Check sheet for the modelled part. Datum: model origin and axes. Units: mm. A direction names the side the tool comes from. Coordinates: 2 decimals unless noted, no trailing zeros. Write each loop counter-clockwise with the first axis right and the second up, starting at its lowest first coordinate (ties: lowest second). Pieces come first, ordered by that corner, then holes. Notation, with made-up numbers: (81.25, 45) -> (138.25, 45) arc R13 cw to (138.25, 62) -> close; hole circle Ø7 at (-18, 47). An arc over 180 degrees is marked (long way). Put each result on its own line as item: value.
```python
from build123d import *

# Parameters (mm, degrees)
BOSS_EXTRUDE1_DEPTH = 6
SKETCH2_W           = 6
SKETCH2_H           = 25.4
SKETCH2_W_2         = 31.8008
SKETCH2_H_2         = 3.048
BOSS_EXTRUDE4_DEPTH = 6
FILLET1_R           = 3.175
KERF_DEPTH          = 6


with BuildPart() as part:
    # Sketch1 → Boss-Extrude1 (new body)
    with BuildSketch(Plane(origin=(0, 0, 0), x_dir=(1, 0, 0), z_dir=(0, 1, 0))):
        Polygon((-3.175, 76.2), (-3.175, -76.2), (57.15, -76.2), (0, 76.2), align=None)
    extrude(amount=BOSS_EXTRUDE1_DEPTH)

    # Sketch2 → Boss-Extrude4 (add)
    with BuildSketch(Plane(origin=(0, 0, 0), x_dir=(1, 0, 0), z_dir=(0, 1, 0))):
        with Locations((-6.175, 0)):
            Rectangle(SKETCH2_W, SKETCH2_H)
        with Locations((-6.175, 38.1)):
            Rectangle(SKETCH2_W, SKETCH2_H)
        with Locations((-6.175, -38.1)):
            Rectangle(SKETCH2_W, SKETCH2_H)
        with Locations((25.4, -77.724)):
            Rectangle(SKETCH2_W_2, SKETCH2_H_2)
    extrude(amount=BOSS_EXTRUDE4_DEPTH)

    # Fillet1
    fillet1_edges = [part.edges().sort_by_distance(p)[0] for p in [
        (0, 3, -76.2),
        (57.15, 3, 76.2),
    ]]
    fillet(fillet1_edges, radius=FILLET1_R)

    # Sketch3 → KERF (add)
    with BuildSketch(Plane(origin=(0, 6, 0), x_dir=(1, 0, 0), z_dir=(0, 1, 0))):
        with BuildLine():
            Line((41.402, -76.3016), (52.568473514, -76.3016))
            ThreePointArc((52.568473514, -76.3016), (55.261594992, -74.891334445), (55.636449697, -71.874508931))
            Line((55.636449697, -71.874508931), (0.867699697, 74.175491069))
            ThreePointArc((0.867699697, 74.175491069), (-0.333942041, 75.718121478), (-2.200276486, 76.3016))
            Line((-2.200276486, 76.3016), (-3.2766, 76.3016))
            Line((-3.2766, 76.3016), (-3.2766, 50.9016))
            Line((-3.2766, 50.9016), (-9.2766, 50.9016))
            Line((-9.2766, 50.9016), (-9.2766, 25.2984))
            Line((-9.2766, 25.2984), (-3.2766, 25.2984))
            Line((-3.2766, 25.2984), (-3.2766, 12.8016))
            Line((-3.2766, 12.8016), (-9.2766, 12.8016))
            Line((-9.2766, 12.8016), (-9.2766, -12.8016))
            Line((-9.2766, -12.8016), (-3.2766, -12.8016))
            Line((-3.2766, -12.8016), (-3.2766, -25.2984))
            Line((-3.2766, -25.2984), (-9.2766, -25.2984))
            Line((-9.2766, -25.2984), (-9.2766, -50.9016))
            Line((-9.2766, -50.9016), (-3.2766, -50.9016))
            Line((-3.2766, -50.9016), (-3.2766, -76.3016))
            Line((-3.2766, -76.3016), (9.398, -76.3016))
            Line((9.398, -76.3016), (9.398, -79.3496))
            Line((9.398, -79.3496), (41.402, -79.3496))
            Line((41.402, -79.3496), (41.402, -76.3016))
        make_face()
    extrude(amount=-KERF_DEPTH)


solid = part.part
```
Q1. Tool access check on faces 4 (the flat face through (9.398, 3, 78)), 5 (the cylindrical face through (-0.31, 3.04, -75.7)), 6 (the flat face through (-6, 3, 12.802)), 7 (the flat face through (41.402, 3, 78)). Record the directions out of +Z, -Z, +X, -X, +Y, -Y that give a thin tool (end or side, any length) a straight path to the whole face; none if there is none.
Recorded:
face 4: +Z, -X, +Y, -Y
face 5: -Z, +X, +Y, -Y
face 6: -X, +Y, -Y
face 7: +Z, +X, +Y, -Y
Q2. Mould release check, pull along Z, two halves, no side actions. Record for faces 1 (the flat face through (-3.277, 3, -64)), 2 (the flat face through (47, 3, 76.302)), 3 (the flat face through (-3.277, 3, -19)): released by +Z, released by -Z, zero draft, split by the parting line, or undercut.
Recorded:
face 1: zero draft
face 2: released by +Z
face 3: undercut
Q3. Cross-section at A-A (y = 2.1). Record the cut outline in (x, z) (1 decimal).
Recorded:
outline: (-9.3, -50.9) -> (-3.3, -50.9) -> (-3.3, -76.3) -> (-2.2, -76.3) arc R3.3 ccw to (0.9, -74.2) -> (55.6, 71.9) arc R3.3 ccw to (52.6, 76.3) -> (41.4, 76.3) -> (41.4, 79.3) -> (9.4, 79.3) -> (9.4, 76.3) -> (-3.3, 76.3) -> (-3.3, 50.9) -> (-9.3, 50.9) -> (-9.3, 25.3) -> (-3.3, 25.3) -> (-3.3, 12.8) -> (-9.3, 12.8) -> (-9.3, -12.8) -> (-3.3, -12.8) -> (-3.3, -25.3) -> (-9.3, -25.3) -> close
Q4. Material ranges on line 1 along Z through (x, y) = (-2, 4.8); line 2 along X through (y, z) = (3.95, 58); line 3 along X through (y, z) = (5.4, -36.5), recorded low to high.
Recorded:
line 1: z = -76.3 to 76.3
line 2: x = -3.28 to 50.43
line 3: x = -9.28 to 15
Q5. Cross-section at B-B (z = -18). Record the cut outline in (x, y), plus the area to 3 significant figures.
Recorded:
outline: (-3.28, 0) -> (21.93, 0) -> (21.93, 6) -> (-3.28, 6) -> close
area: 151 mm2
Q6. Depth check by flat-ended pin: P1, Ø2, axis at x = 1.5, y = 2, coming from the -Z side; P2, Ø3, axis at x = -6.5, y = 2.5, coming from the +Z side; P3, Ø2.5, axis at y = 4, z = 77.5, coming from the -X side; P4, Ø12, axis at x = 15.5, z = -53, coming from the +Y side (3 decimals). Enter the tip coordinate at first touch or a pass-through.
Recorded:
P1: stops at z = -74.88
P2: stops at z = 50.9
P3: stops at x = -3.28
P4: passes through
Q7. Cross-section at C-C (x = 7). Record the cut outline in (y, z), plus the area to 3 significant figures.
Recorded:
outline: (0, -57.82) -> (6, -57.82) -> (6, 76.3) -> (0, 76.3) -> close
area: 805 mm2
